Geometry check sheet. Reference: the model listing, model coordinates, mm. Face numbers are marked on the shaded views. A direction names the side the tool comes from. Round coordinates to 2 decimals unless told otherwise and drop trailing zeros. Write each loop counter-clockwise with the first axis right and the second up, starting at its lowest first coordinate (ties: lowest second). Pieces come first, ordered by that corner, then holes. Notation, with made-up numbers: (49, -15) - (61, -15) arc R18 ccw to (61, 18) - close; hole circle Ø5 at (49, -18.5). An arc over 180 degrees is marked (long way). Return JSON: item names as keys, results as strings.
```python
from build123d import *

# Parameters (mm, degrees)
SKETCH1_R           = 1.5
BOSS_EXTRUDE1_DEPTH = 3
SKETCH3_W           = 4.615398666
SKETCH3_H           = 10
BOSS_EXTRUDE2_DEPTH = 12.9997796
FILLET7_R           = 1
CUT_EXTRUDE4_DEPTH  = 10
FILLET8_R           = 4
SKETCH8_W           = 76
SKETCH8_H           = 10
BOSS_EXTRUDE3_DEPTH = 4.615398666
SKETCH9_W           = 14.615398666
SKETCH9_H           = 12
SKETCH9_R           = 1.5
BOSS_EXTRUDE4_DEPTH = 3
FILLET9_R           = 5
FILLET10_R          = 5
SKETCH10_W          = 9.773230982
SKETCH10_H          = 9.985016007
SKETCH10_W_2        = 12.713773796
SKETCH10_H_2        = 7.76031956
CUT_EXTRUDE6_DEPTH  = 10


with BuildPart() as part:
    # Sketch1 → Boss-Extrude1 (new body)
    with BuildSketch(Plane(origin=(0, 0, 0), x_dir=(1, 0, 0), z_dir=(0, 1, 0))):
        Polygon((-3, -11.32792047), (3, -11.32792047), (3, -5), (7.615398666, -5), (7.615398666, 5), (3, 5), (3, 11.32792047), (-3, 11.32792047), align=None)
        with Locations(Location((0, 8.5, 0), (0, 0, 270))):
            Circle(SKETCH1_R, mode=Mode.SUBTRACT)
        with Locations(Location((0, -8.5, 0), (0, 0, 270))):
            Circle(SKETCH1_R, mode=Mode.SUBTRACT)
    extrude(amount=BOSS_EXTRUDE1_DEPTH)

    # Sketch3 → Boss-Extrude2 (add)
    with BuildSketch(Plane(origin=(0, 3, 0), x_dir=(1, 0, 0), z_dir=(0, 1, 0))):
        with Locations((5.307699333, 0)):
            Rectangle(SKETCH3_W, SKETCH3_H)
    extrude(amount=BOSS_EXTRUDE2_DEPTH)

    # Fillet7
    fillet7_edges = [part.edges().sort_by_distance(p)[0] for p in [
        (3, 1.5, 11.32792047),
        (3, 1.5, -11.32792047),
    ]]
    fillet(fillet7_edges, radius=FILLET7_R)

    # Sketch7 → Cut-Extrude4 (cut)
    with BuildSketch(Plane.XZ):
        with BuildLine():
            Line((-3.65526474, -6.392053518), (-3.78188192, 6.478485425))
            ThreePointArc((-3.78188192, 6.478485425), (-0.319780446, 0.076652438), (-3.65526474, -6.392053518))
        make_face()
    extrude(amount=-CUT_EXTRUDE4_DEPTH, mode=Mode.SUBTRACT)

    # Fillet8
    fillet8_edges = [part.edges().sort_by_distance(p)[0] for p in [
        (3, 3, 0),
    ]]
    fillet(fillet8_edges, radius=FILLET8_R)

    # Sketch8 → Boss-Extrude3 (add)
    with BuildSketch(Plane(origin=(7.615398666, 0, 0), x_dir=(0, 0, -1), z_dir=(1, 0, 0))):
        with Locations((0, 10.9997796)):
            Rectangle(SKETCH8_W, SKETCH8_H)
    extrude(amount=-BOSS_EXTRUDE3_DEPTH)

    # Sketch9 → Boss-Extrude4 (add)
    # profile 1 of 2: a face of its own
    with BuildSketch(Plane(origin=(0, 15.9997796, 0), x_dir=(1, 0, 0), z_dir=(0, 1, 0))):
        with Locations((10.307699333, 32)):
            Rectangle(SKETCH9_W, SKETCH9_H)
        with Locations(Location((12.745112207, 32.5, 0), (0, 0, 270))):
            Circle(SKETCH9_R, mode=Mode.SUBTRACT)
    # profile 2 of 2: a face of its own
    with BuildSketch(Plane(origin=(0, 15.9997796, 0), x_dir=(1, 0, 0), z_dir=(0, 1, 0))):
        with Locations((10.307699333, -32)):
            Rectangle(SKETCH9_W, SKETCH9_H)
        with Locations(Location((12.745112207, -32.5, 0), (0, 0, 270))):
            Circle(SKETCH9_R, mode=Mode.SUBTRACT)
    extrude(amount=BOSS_EXTRUDE4_DEPTH)

    # Fillet9
    # the kernel refuses this fillet: 5 mm, written as the material it adds along each edge
    with BuildSketch(Plane(origin=(7.615398666, 5.9997796, 5), x_dir=(0, -1, 0), z_dir=(-1, 0, 0))) as fillet9_piece_1:
        with BuildLine():
            CenterArc((FILLET9_R, FILLET9_R), FILLET9_R, 180, 90)
            Line((0, FILLET9_R), (0, 0))
            Line((0, 0), (FILLET9_R, 0))
        make_face()
    extrude(amount=4.615398666)

    # Fillet10
    # the kernel refuses this fillet: 5 mm, written as the material it adds along each edge
    with BuildSketch(Plane(origin=(3, 5.9997796, -5), x_dir=(0, -1, 0), z_dir=(1, 0, 0))) as fillet10_piece_1:
        with BuildLine():
            CenterArc((FILLET10_R, FILLET10_R), FILLET10_R, 180, 90)
            Line((0, FILLET10_R), (0, 0))
            Line((0, 0), (FILLET10_R, 0))
        make_face()
    extrude(amount=4.615398666)

    # Sketch10 → Cut-Extrude6 (cut)
    with BuildSketch(Plane(origin=(0, 3, 0), x_dir=(1, 0, 0), z_dir=(0, 1, 0))):
        with Locations((-1.330252474, 10.872508004)):
            Rectangle(SKETCH10_W, SKETCH10_H)
        with Locations((-2.800523881, -9.76015978)):
            Rectangle(SKETCH10_W_2, SKETCH10_H_2)
    extrude(amount=-CUT_EXTRUDE6_DEPTH, mode=Mode.SUBTRACT)


solid = part.part
```
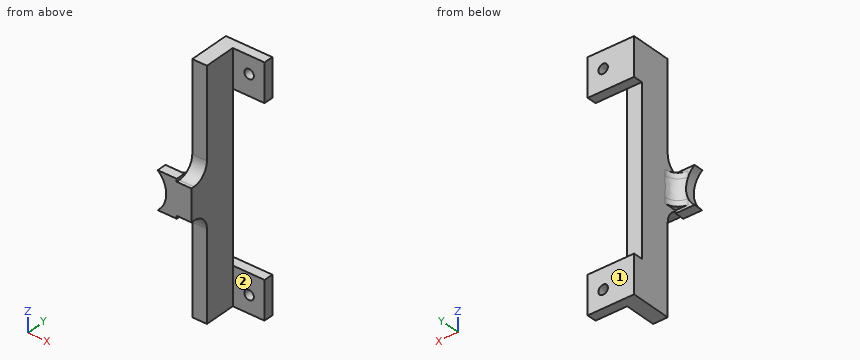
(1) Section check A-A, the plane z = 32.5. Enter the section's corners in (x, y).
Response values:
{"outline": "(3, 6) - (7.62, 6) - (7.62, 16) - (11.25, 16) - (11.25, 19) - (3, 19) - close; (14.25, 16) - (17.62, 16) - (17.62, 19) - (14.25, 19) - close"}
(2) Gauge pin test, flat ends, axial feed: pin 1 (4 mm diameter, centred on x = 12.75, z = 32.5, fed in from -Y); pin 2 (1.3 mm diameter, centred on x = 0.5, z = -5, fed in from +Y); pin 3 (5 mm diameter, centred on x = 7.5, z = -21.5, fed in from +Y). Record the tip position at first contact, or that the pin passes through.
Response values:
{"pin 1": "stops at y = 16", "pin 2": "stops at y = 3.63", "pin 3": "stops at y = 16"}
(3) Section check D-D, the plane y = 12.25. Enter the section's corners in (x, z).
Response values:
{"outline": "(3, -38) - (7.62, -38) - (7.62, 38) - (3, 38) - close"}
(4) Material ranges on line 1 along Z through (x, y) = (5, 16.5); line 2 along X through (y, z) = (18.1, -32.5); line 3 along X through (y, z) = (11.5, 33), recorded low to high. Write a range as [from, to].
Response values:
{"line 1": "z = [-38, -26], [26, 38]", "line 2": "x = [3, 11.25], [14.25, 17.62]", "line 3": "x = [3, 7.62]"}
(5) Section check B-B, the plane y = 18.25. Enter the section's corners in (x, z).
Response values:
{"outline": "(3, -38) - (17.62, -38) - (17.62, -26) - (3, -26) - close; (3, 26) - (17.62, 26) - (17.62, 38) - (3, 38) - close; hole circle Ø3 at (12.75, -32.5); hole circle Ø3 at (12.75, 32.5)"}
(6) Section check C-C, the plane x = 5.5. Enter the section's corners in (y, z), plus the area to 3 significant figures.
Response values:
{"outline": "(0, -5) - (1, -5) arc R5 cw to (6, -10) - (6, -38) - (19, -38) - (19, -26) - (16, -26) - (16, 26) - (19, 26) - (19, 38) - (6, 38) - (6, 10) arc R5 cw to (1, 5) - (0, 5) - close", "area": "903 mm^2"}
(7) Access from +Z, -Z, +X, -X, +Y, -Y to the whole of each face (thin tool, end or side, straight path). Record for the marked faces 1 and 2.
Response values:
{"face 1": "+Z, -Z, +X, -X, +Y", "face 2": "+Z, -Z, +X, -Y"}
